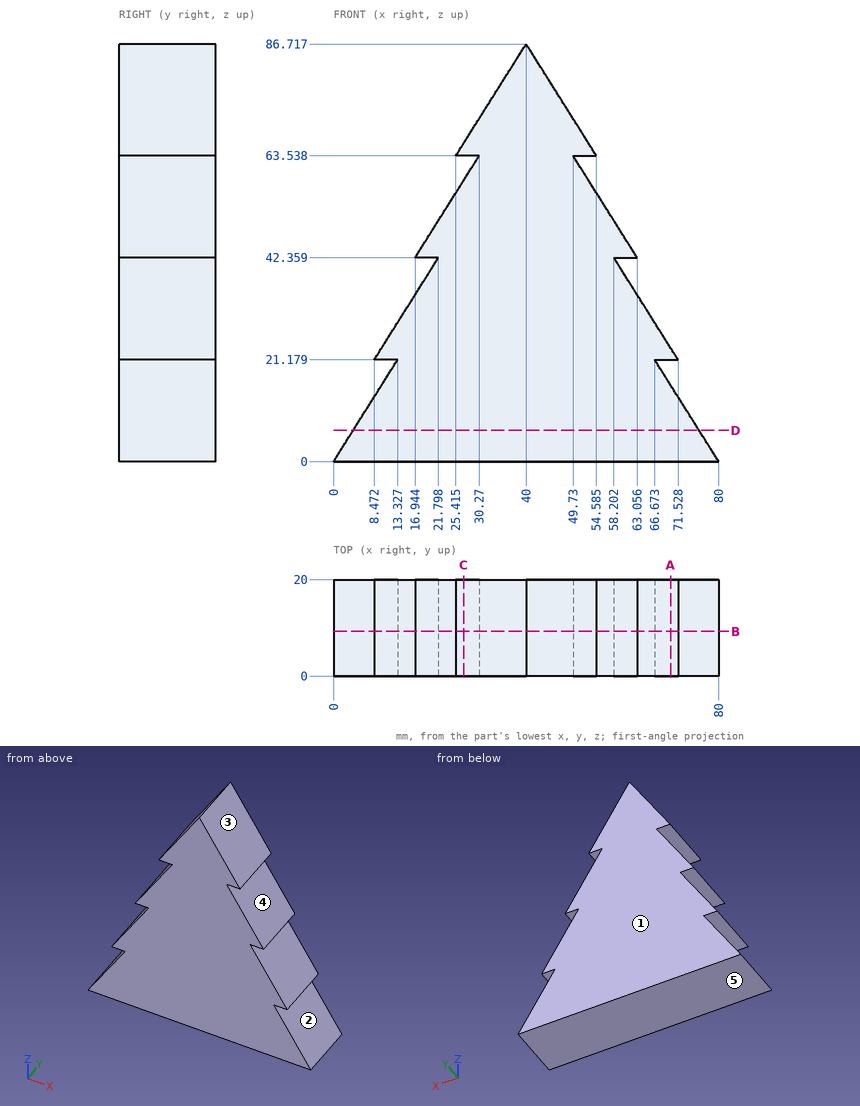
Geometry check sheet. Reference: drawing and pictorial views, mm from the part's lowest x, y, z. A direction names the side the tool comes from. Give positions to 0.01 mm unless a question says otherwise; leave off trailing zeros. Write each loop counter-clockwise with the first axis right and the second up, starting at its lowest first coordinate (ties: lowest second). Pieces come first, ordered by that corner, then holes. Notation, with made-up numbers: (-25.75, 37) - (11.25, 37) arc R12 cw to (11.25, 57) - close; hole circle Ø1 at (34, 30.5). An arc over 180 degrees is marked (long way). Put each result on its own line as item: value.
Q1. Section check B-B on y = 9.25. Record the cut outline in (x, z) (1 decimal).
Result:
outline: (0, 0) - (80, 0) - (66.7, 21.2) - (71.5, 21.2) - (58.2, 42.4) - (63.1, 42.4) - (49.7, 63.5) - (54.6, 63.5) - (40, 86.7) - (25.4, 63.5) - (30.3, 63.5) - (16.9, 42.4) - (21.8, 42.4) - (8.5, 21.2) - (13.3, 21.2) - close
Q2. Section check C-C on x = 27. Record the cut outline in (y, z), and give its area (3 significant figures).
Result:
outline: (0, 0) - (20, 0) - (20, 58.34) - (0, 58.34) - close; (0, 63.54) - (20, 63.54) - (20, 66.06) - (0, 66.06) - close
area: 1,220 mm2
Q3. Section check A-A on x = 70. Record the cut outline in (y, z).
Result:
outline: (0, 0) - (20, 0) - (20, 15.89) - (0, 15.89) - close; (0, 21.18) - (20, 21.18) - (20, 23.61) - (0, 23.61) - close
Q4. Scan lines: probe 1 along Z at (x, y) = (28, 9.75) (1 decimal); probe 2 along Z at (x, y) = (62, 16) (1 decimal); probe 3 along X at (y, z) = (5.5, 20) (1 decimal). Record each from-to range of solid material in increasing order. Write a range as from..to.
Result:
probe 1: 0..59.9, 63.5..67.6
probe 2: 0..36.3, 42.4..44
probe 3: 12.6..67.4
Q5. Mould release check, pull along Z, two halves, no side actions. Record for the marked faces 1, 2 and 3: released by +Z, released by -Z, zero draft, split by the parting line, or undercut.
Result:
face 1: zero draft
face 2: undercut
face 3: released by +Z
Q6. Section check D-D on z = 6.5. Record the cut outline in (x, y), and give its area (3 significant figures).
Result:
outline: (4.09, 0) - (75.91, 0) - (75.91, 20) - (4.09, 20) - close
area: 1,440 mm2
Q7. Depth check by flat-ended pin: P1, Ø3, axis at x = 58.5, y = 9.5, coming from the +Z side (1 decimal); P2, Ø6, axis at y = 16, z = 19, coming from the +X side; P3, Ø5, axis at y = 12, z = 30.5, coming from the +X side. Enter the tip coordinate at first touch or a pass-through.
Result:
P1: z = 52
P2: x = 71.53
P3: x = 67.24
Q8. Set-up check for the marked faces 4 and 5: record each of +Z, -Z, +X, -X, +Y, -Y from which the full face is reachable in a straight line by a thin tool's end or side.
Result:
face 4: +X, +Y, -Y
face 5: -Z, +X, -X, +Y, -Y
